from build123d import *

# Parameters (mm, degrees)
SKETCH_1_R      = 5
EXTRUDE_2_DEPTH = 5
EXTRUDE_4_DEPTH = 15
EXTRUDE_5_DEPTH = 20


with BuildPart() as part:
    # Sketch 1 → Extrude 2 (new body)
    with BuildSketch(Plane(origin=(0, 0, 0), x_dir=(1, 0, 0), z_dir=(0, 1, 0))):
        with BuildLine():
            Line((0, -10), (-15, -10))
            Line((-15, -10), (-15, 10))
            Line((-15, 10), (0, 10))
            ThreePointArc((0, 10), (10, 0), (0, -10))
        make_face()
        Circle(SKETCH_1_R, mode=Mode.SUBTRACT)
    extrude(amount=EXTRUDE_2_DEPTH)

    # Sketch 1_4 → Extrude 4 (add)
    with BuildSketch(Plane(origin=(0, 0, 0), x_dir=(1, 0, 0), z_dir=(0, 1, 0))):
        with BuildLine():
            Line((-5, 0), (-5, -10))
            Line((-5, -10), (0, -10))
            Line((0, -10), (0, -5))
            ThreePointArc((0, -5), (-3.535533906, -3.535533906), (-5, 0))
        make_face()
        with BuildLine():
            Line((-5, 10), (-5, 0))
            ThreePointArc((-5, 0), (-3.535533906, 3.535533906), (0, 5))
            Line((0, 5), (0, 10))
            Line((0, 10), (-5, 10))
        make_face()
        Polygon((-15, -10), (-5, -10), (-5, 0), (-5, 10), (-15, 10), align=None)
    extrude(amount=EXTRUDE_4_DEPTH)

    # Sketch 1_5 → Extrude 5 (add)
    with BuildSketch(Plane(origin=(0, 0, 0), x_dir=(1, 0, 0), z_dir=(0, 1, 0))):
        Polygon((-15, -10), (-5, -10), (-5, 0), (-5, 10), (-15, 10), align=None)
    extrude(amount=EXTRUDE_5_DEPTH)


solid = part.part
Verification items for the finished model (mm, model axes). A direction names the side the tool comes from. Coordinates: 2 decimals unless noted, no trailing zeros. Write each loop counter-clockwise with the first axis right and the second up, starting at its lowest first coordinate (ties: lowest second). Pieces come first, ordered by that corner, then holes. Notation, with made-up numbers: (76.5, 87.5) -> (124.5, 87.5) arc R9 cw to (124.5, 102.5) -> close; hole circle Ø10 at (23.5, 67). An arc over 180 degrees is marked (long way). One line per item, written item: value. Start each with the question number.
Q1. Go/stop test with flat-tipped pins: P1, Ø1.5, axis at y = 11.5, z = 7, coming from the +X side; P2, Ø5.5, axis at x = -2, z = 3.5, coming from the +Y side; P3, Ø5.5, axis at y = 18, z = -1.5, coming from the +X side; P4, Ø1, axis at x = -2.5, y = 16, coming from the -Z side. Record where each tip stops, or that it passes through.
Q2. Cross-section at D-D on y = 5.5. Enter the section's corners in (x, z), and give its area (3 significant figures).
Q3. Thickness scan on L1, parallel to X at y = 16, z = 0; L2, parallel to X at y = 7.75, z = 6; L3, parallel to Y at x = -1, z = 8.5. Record the ranges inside material, lowest first. Write a range as from..to.
Q4. Cross-section at B-B on z = 2.5. Enter the section's corners in (x, y).
Q5. Cross-section at A-A on y = 1.75. Enter the section's corners in (x, z), and give its area (3 significant figures).
Q6. Access from +Z, -Z, +X, -X, +Y, -Y to the whole of each face (thin tool, end or side, straight path). Record for faces 1 (the flat face through (0, 10, 8)), 2 (the flat face through (-10, 20, 0)).
Q7. Cross-section at C-C on x = -0.75. Enter the section's corners in (y, z).
Checked values:
1. P1: stops at x = 0
1. P2: stops at y = 15
1. P3: stops at x = -5
1. P4: passes through
2. outline: (-15, -10) -> (0, -10) -> (0, -5) arc R5 cw to (0, 5) -> (0, 10) -> (-15, 10) -> close
2. area: 261 mm²
3. L1: x = -15..-5
3. L2: x = -15..0
3. L3: y = 0..15
4. outline: (-15, 0) -> (-4.33, 0) -> (-4.33, 15) -> (-5, 15) -> (-5, 20) -> (-15, 20) -> close; (4.33, 0) -> (9.68, 0) -> (9.68, 5) -> (4.33, 5) -> close
5. outline: (-15, -10) -> (0, -10) arc R10 ccw to (0, 10) -> (-15, 10) -> close; hole circle Ø10 at (0, 0)
5. area: 379 mm²
6. face 1: +Z, -Z, +X, +Y
6. face 2: +Z, -Z, +X, -X, +Y
7. outline: (0, -10) -> (15, -10) -> (15, -4.94) -> (0, -4.94) -> close; (0, 4.94) -> (15, 4.94) -> (15, 10) -> (0, 10) -> close
